Autodesk Inventor part; units mm, degrees
ref_plane "YZ Plane" through (0, 0, 0) normal (1, 0, 0) x (0, 1, 0)
ref_plane "XZ Plane" through (0, 0, 0) normal (0, 1, 0) x (-1, 0, 0)
ref_plane "XY Plane" through (0, 0, 0) normal (0, 0, 1) x (1, 0, 0)
sketch "Sketch1" plane through (0, 0, 0) normal (0, 0, 1) x (1, 0, 0)
  line L0 (0, 0) -> (20, 0)
  line L1 (20, 0) -> (20, 25)
  line L2 (20, 25) -> (15, 25)
  line L3 (15, 25) -> (15, 10)
  line L4 (10, 5) -> (10, 5)
  line L5 (5, 10) -> (5, 25)
  line L6 (5, 25) -> (0, 25)
  line L7 (0, 25) -> (0, 0)
  arc A0 (5, 10) -> (10, 5) centre (10, 10) ccw
  arc A1 (10, 5) -> (15, 10) centre (10, 10) ccw
  point P0 (15, 5)
  point P1 (5, 5)
  dimension "d0" = 20
  dimension "d1" = 25
  dimension "d2" = 5
  dimension "d3" = 20
  dimension "d4" = 10
  dimension "d5" = 5
extrude "Extrusion1" add sketch "Sketch1" against normal blind 5
sketch "Sketch2" plane through (0, 0, -5) normal (0, 0, -1) x (-1, 0, 0)
  line L0 (0, 25) -> (0, 0)
  line L1 (-20, 25) -> (-20, 0)
  line L2 (0, 0) -> (-20, 0)
  line L3 (-20, 0) -> (-20, 5)
  line L4 (-20, 5) -> (0, 5)
  line L5 (0, 5) -> (0, 0)
  dimension "d8" = 5
extrude "Extrusion2" add sketch "Sketch2" along normal blind 15
sketch "Sketch3" plane through (0, 0, -20) normal (0, 0, -1) x (-1, 0, 0)
  line L0 (-20, 25) -> (-20, 5)
  line L1 (0, 0) -> (-20, 0)
  line L2 (-20, 0) -> (-20, 15)
  line L3 (-10, 25) -> (-10, 25)
  line L4 (0, 15) -> (0, 0)
  arc A0 (-10, 25) -> (-20, 15) centre (-10, 15) ccw
  arc A1 (0, 15) -> (-10, 25) centre (-10, 15) ccw
  circle A2 centre (-10, 15) radius 5
  dimension "d11" = 10
  dimension "d12" = 10
extrude "Extrusion3" add sketch "Sketch3" against normal blind 5
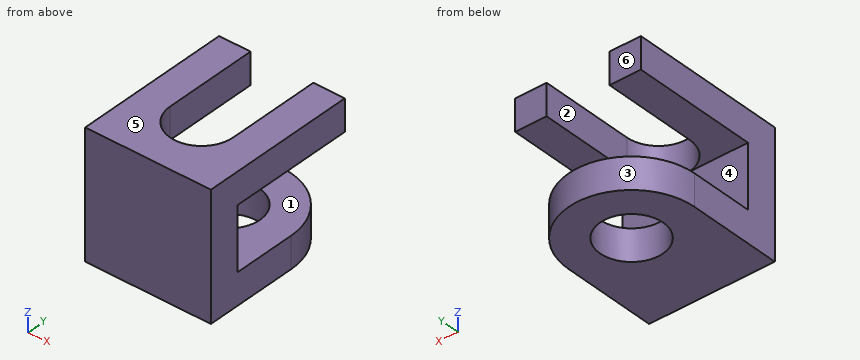
Model file for the job. Use its own axes, mm. Face numbers are marked on the shaded views. A direction names the side the tool comes from. Coordinates: 2 decimals unless noted, no trailing zeros. Loops run counter-clockwise (first coordinate to the right, second up) from the corner with the lowest first, then second, coordinate; pieces in that order, holes last. Notation, with made-up numbers: M 64.25,7 L 118.25,7 A36 ccw 118.25,41 Z; hole C 39.5,-28.75 d1. An arc over 180 degrees is marked long. Use CSV: the item, a comma, the result in double quotes. Start each with the question number.
1. Flat gauge pins, fed straight in: pin 1 (11 mm diameter, centred on x = 13.5, z = -10.5, fed in from +Y); pin 2 (1 mm diameter, centred on x = 7, y = 7.5, fed in from +Z). Where does each tip first touch, or does it go through?
2. Tool access for the marked faces 1, 2 and 3: list every direction of +Z, -Z, +X, -X, +Y, -Y with a clear straight run to the whole face (end or side of a thin tool).
3. Probe probe 1 along Z at (x, y) = (16, 9.5); probe 2 along Y at (x, z) = (10, -17.75); probe 3 along X at (y, z) = (11.75, -1). List the from-to ranges inside material, lowest first. Write a range as [from, to].
4. Band-saw the part on B-B, the plane x = 6.25. List the corners of the cut face in (y, z).
5. Band-saw the part on D-D, the plane y = 9. List the corners of the cut face in (x, z), then the cut area to 3 significant figures.
6. Band-saw the part on C-C, the plane z = -18. List the corners of the cut face in (x, y), then the cut area to 3 significant figures.
7. Band-saw the part on A-A, the plane y = 15.75. List the corners of the cut face in (x, z).
8. Two-plate mould, pull along Z, no slides. Class the marked faces 4, 5 and 6: pulls with the +Z half, pulls with the -Z half, needs draft (parallel to the pull), parting line crosses it, or undercut.
Entries:
1,pin 1,"stops at y = 24.99"
1,pin 2,"stops at z = -15"
2,face 1,"+X, -X, +Y"
2,face 2,"+Z, +Y"
2,face 3,"-Z, +Y"
3,probe 1,"z = [-20, -15], [-5, 0]"
3,probe 2,"y = [0, 10], [20, 25]"
3,probe 3,"x = [0, 5], [15, 20]"
4,outline,"M 0,-20 L 11.69,-20 L 11.69,-15 L 5,-15 L 5,-5 L 6.69,-5 L 6.69,0 L 0,0 Z; M 18.31,-20 L 24.27,-20 L 24.27,-15 L 18.31,-15 Z"
5,outline,"M 0,-20 L 20,-20 L 20,-15 L 0,-15 Z; M 0,-5 L 5.1,-5 L 5.1,0 L 0,0 Z; M 14.9,-5 L 20,-5 L 20,0 L 14.9,0 Z"
5,area,"151 mm2"
6,outline,"M 0,0 L 20,0 L 20,15 A10 ccw 0,15 Z; hole C 10,15 d10"
6,area,"379 mm2"
7,outline,"M 0,-5 L 5,-5 L 5,0 L 0,0 Z; M 0.03,-20 L 5.06,-20 L 5.06,-15 L 0.03,-15 Z; M 14.94,-20 L 19.97,-20 L 19.97,-15 L 14.94,-15 Z; M 15,-5 L 20,-5 L 20,0 L 15,0 Z"
8,face 4,"undercut"
8,face 5,"pulls with the +Z half"
8,face 6,"needs draft"
